Here's how the part is built. I have some questions about the finished solid (model axes, mm). Round coordinates to 2 decimals unless told otherwise and drop trailing zeros. Loops run counter-clockwise (first coordinate to the right, second up) from the corner with the lowest first, then second, coordinate; pieces in that order, holes last. Notation, with made-up numbers: M 10.5,-2.5 L 43.5,-2.5 A15 ccw 43.5,4.5 Z; hole C 75,17 d1. An arc over 180 degrees is marked long. Use a Markdown table: item, result.
```python
from build123d import *

# Parameters (mm, degrees)
SKETCH2_R           = 1
SKETCH2_R_2         = 3
BOSS_EXTRUDE2_DEPTH = 4.7625


with BuildPart() as part:
    # Sketch2 → Boss-Extrude2 (new body)
    # profile 1 of 7: a face of its own
    with BuildSketch(Plane(origin=(0, 0, 0), x_dir=(1, 0, 0), z_dir=(0, 1, 0))):
        with BuildLine():
            Line((0, 32), (0, 30))
            ThreePointArc((0, 30), (21.213203436, 21.213203436), (30, 0))
            Line((30, 0), (33.432819775, 0))
            ThreePointArc((33.432819775, 0), (33.386867146, 5.204755795), (37.902132901, 2.615553276))
            ThreePointArc((37.902132901, 2.615553276), (37.491335421, 1.10028752), (36.371446028, 0))
            Line((36.371446028, 0), (48, 0))
            ThreePointArc((48, 0), (33.941125497, 33.941125497), (0, 48))
            Line((0, 48), (0, 38))
            ThreePointArc((0, 38), (2.121320344, 37.121320344), (3, 35))
            ThreePointArc((3, 35), (2.121320344, 32.878679656), (0, 32))
        make_face()
        with Locations(Location((42.896828136, 9.790921094, 0), (0, 0, 90))):
            Circle(SKETCH2_R, mode=Mode.SUBTRACT)
        with Locations(Location((32.580581203, 12.786935853, 0), (0, 0, 90))):
            Circle(SKETCH2_R_2, mode=Mode.SUBTRACT)
        with Locations(Location((27.364101886, 21.822143065, 0), (0, 0, 90))):
            Circle(SKETCH2_R_2, mode=Mode.SUBTRACT)
        with Locations(Location((10.316431104, 33.445048203, 0), (0, 0, 90))):
            Circle(SKETCH2_R_2, mode=Mode.SUBTRACT)
        with Locations(Location((19.716202032, 28.918357101, 0), (0, 0, 90))):
            Circle(SKETCH2_R_2, mode=Mode.SUBTRACT)
        with Locations(Location((19.090884521, 39.642630188, 0), (0, 0, 90))):
            Circle(SKETCH2_R, mode=Mode.SUBTRACT)
    # profile 2 of 7: a face of its own
    with BuildSketch(Plane(origin=(0, 0, 0), x_dir=(1, 0, 0), z_dir=(0, 1, 0))):
        with BuildLine():
            Line((33.432819775, 0), (30, 0))
            ThreePointArc((30, 0), (0, -30), (-30, 0))
            Line((-30, 0), (-33.432819775, 0))
            ThreePointArc((-33.432819775, 0), (-34.902132901, -0.384446724), (-36.371446028, 0))
            Line((-36.371446028, 0), (-48, 0))
            ThreePointArc((-48, 0), (-44.712414383, -17.458522274), (-35.3, -32.525528435))
            ThreePointArc((-35.3, -32.525528435), (-19.271411924, -43.961490903), (0, -48))
            ThreePointArc((0, -48), (19.271411924, -43.961490903), (35.3, -32.525528435))
            ThreePointArc((35.3, -32.525528435), (44.712414383, -17.458522274), (48, 0))
            Line((48, 0), (36.371446028, 0))
            ThreePointArc((36.371446028, 0), (34.902132901, -0.384446724), (33.432819775, 0))
        make_face()
        with Locations(Location((-34.400585229, -27.433551282, 0), (0, 0, 90))):
            Circle(SKETCH2_R, mode=Mode.SUBTRACT)
        with Locations(Location((-15.185930869, -31.533910377, 0), (0, 0, 90))):
            Circle(SKETCH2_R_2, mode=Mode.SUBTRACT)
        with Locations(Location((-23.806045822, -25.656815514, 0), (0, 0, 90))):
            Circle(SKETCH2_R_2, mode=Mode.SUBTRACT)
        with Locations(Location((-5.216479316, -34.609078918, 0), (0, 0, 90))):
            Circle(SKETCH2_R_2, mode=Mode.SUBTRACT)
        with Locations(Location((-30.310889132, -17.5, 0), (0, 0, 90))):
            Circle(SKETCH2_R_2, mode=Mode.SUBTRACT)
        with Locations(Location((-34.122476926, -7.788232688, 0), (0, 0, 90))):
            Circle(SKETCH2_R_2, mode=Mode.SUBTRACT)
        with Locations(Location((0, -44, 0), (0, 0, 90))):
            Circle(SKETCH2_R, mode=Mode.SUBTRACT)
        with Locations(Location((5.216479316, -34.609078918, 0), (0, 0, 90))):
            Circle(SKETCH2_R_2, mode=Mode.SUBTRACT)
        with Locations(Location((15.185930869, -31.533910377, 0), (0, 0, 90))):
            Circle(SKETCH2_R_2, mode=Mode.SUBTRACT)
        with Locations(Location((23.806045822, -25.656815514, 0), (0, 0, 90))):
            Circle(SKETCH2_R_2, mode=Mode.SUBTRACT)
        with Locations(Location((34.400585229, -27.433551282, 0), (0, 0, 90))):
            Circle(SKETCH2_R, mode=Mode.SUBTRACT)
        with Locations(Location((30.310889132, -17.5, 0), (0, 0, 90))):
            Circle(SKETCH2_R_2, mode=Mode.SUBTRACT)
        with Locations(Location((34.122476926, -7.788232688, 0), (0, 0, 90))):
            Circle(SKETCH2_R_2, mode=Mode.SUBTRACT)
    # profile 3 of 7: a face of its own
    with BuildSketch(Plane(origin=(0, 0, 0), x_dir=(1, 0, 0), z_dir=(0, 1, 0))):
        with BuildLine():
            Line((48, -32.525528435), (48, 0))
            ThreePointArc((48, 0), (44.712414383, -17.458522274), (35.3, -32.525528435))
            Line((35.3, -32.525528435), (48, -32.525528435))
        make_face()
    # profile 4 of 7: a face of its own
    with BuildSketch(Plane(origin=(0, 0, 0), x_dir=(1, 0, 0), z_dir=(0, 1, 0))):
        with BuildLine():
            Line((35.3, -48), (35.3, -32.525528435))
            ThreePointArc((35.3, -32.525528435), (19.271411924, -43.961490903), (0, -48))
            Line((0, -48), (35.3, -48))
        make_face()
    # profile 5 of 7: a face of its own
    with BuildSketch(Plane(origin=(0, 0, 0), x_dir=(1, 0, 0), z_dir=(0, 1, 0))):
        with BuildLine():
            ThreePointArc((0, -48), (-19.271411924, -43.961490903), (-35.3, -32.525528435))
            Line((-35.3, -32.525528435), (-35.3, -48))
            Line((-35.3, -48), (0, -48))
        make_face()
    # profile 6 of 7: a face of its own
    with BuildSketch(Plane(origin=(0, 0, 0), x_dir=(1, 0, 0), z_dir=(0, 1, 0))):
        with BuildLine():
            ThreePointArc((-35.3, -32.525528435), (-44.712414383, -17.458522274), (-48, 0))
            Line((-48, 0), (-48, -32.525528435))
            Line((-48, -32.525528435), (-35.3, -32.525528435))
        make_face()
    # profile 7 of 7: a face of its own
    with BuildSketch(Plane(origin=(0, 0, 0), x_dir=(1, 0, 0), z_dir=(0, 1, 0))):
        with BuildLine():
            ThreePointArc((-30, 0), (-21.213203436, 21.213203436), (0, 30))
            Line((0, 30), (0, 32))
            ThreePointArc((0, 32), (-3, 35), (0, 38))
            Line((0, 38), (0, 48))
            ThreePointArc((0, 48), (-33.941125497, 33.941125497), (-48, 0))
            Line((-48, 0), (-36.371446028, 0))
            ThreePointArc((-36.371446028, 0), (-36.417398657, 5.204755795), (-31.902132901, 2.615553276))
            ThreePointArc((-31.902132901, 2.615553276), (-32.312930381, 1.10028752), (-33.432819775, 0))
            Line((-33.432819775, 0), (-30, 0))
        make_face()
        with Locations(Location((-42.896828136, 9.790921094, 0), (0, 0, 90))):
            Circle(SKETCH2_R, mode=Mode.SUBTRACT)
        with Locations(Location((-32.580581203, 12.786935853, 0), (0, 0, 90))):
            Circle(SKETCH2_R_2, mode=Mode.SUBTRACT)
        with Locations(Location((-27.364101886, 21.822143065, 0), (0, 0, 90))):
            Circle(SKETCH2_R_2, mode=Mode.SUBTRACT)
        with Locations(Location((-19.716202032, 28.918357101, 0), (0, 0, 90))):
            Circle(SKETCH2_R_2, mode=Mode.SUBTRACT)
        with Locations(Location((-10.316431104, 33.445048203, 0), (0, 0, 90))):
            Circle(SKETCH2_R_2, mode=Mode.SUBTRACT)
        with Locations(Location((-19.090884521, 39.642630188, 0), (0, 0, 90))):
            Circle(SKETCH2_R, mode=Mode.SUBTRACT)
    extrude(amount=BOSS_EXTRUDE2_DEPTH)


solid = part.part
```
Q1. Will these pins go through, and if not, where does the flat tip stop? P1, Ø2.5, axis at x = -42, y = 1.5, coming from the +Z side; P2, Ø2, axis at y = 3.5, z = -29, coming from the +X side.
Return value:
| item | result |
|---|---|
| P1 | stops at z = 32.53 |
| P2 | stops at x = 38.99 |
Q2. Imagine slicing it at B-B, the plane z = -23. Please give me the cut outline in (x, y) (1 decimal).
Return value:
| item | result |
|---|---|
| outline | M -42.1,0 L -30.1,0 L -30.1,4.8 L -42.1,4.8 Z; M -24.6,0 L -19.3,0 L -19.3,4.8 L -24.6,4.8 Z; M 19.3,0 L 24.6,0 L 24.6,4.8 L 19.3,4.8 Z; M 30.1,0 L 42.1,0 L 42.1,4.8 L 30.1,4.8 Z |
Q3. Imagine slicing it at C-C, the plane y = 1.25. Give the number of separate pieces and of enclosed holes in the cut face, then the cut area to 3 significant figures.
Return value:
| item | result |
|---|---|
| separate pieces | 1 |
| enclosed holes | 29 |
| area | 4,390 mm^2 |
Q4. We'd pull the mould along X, two halves only. Please class faces 1 (the flat face through (-48, 2, 16)), 2 (the flat face through (35.3, 2, 40)), 3 (the cylindrical face through (30.026, 2.348, -23.206)), 4 (the flat face through (42, 2, 32.526)): pulls with the +X half, pulls with the -X half, needs draft (parallel to the pull), parting line crosses it, or undercut.
Return value:
| item | result |
|---|---|
| face 1 | pulls with the -X half |
| face 2 | pulls with the +X half |
| face 3 | undercut |
| face 4 | needs draft |
Q5. Imagine slicing it at A-A, the plane z = 6. Please give me the cut outline in (x, y).
Return value:
| item | result |
|---|---|
| outline | M -48,0 L -36.53,0 L -36.53,4.76 L -48,4.76 Z; M -31.71,0 L -29.39,0 L -29.39,4.76 L -31.71,4.76 Z; M 29.39,0 L 31.71,0 L 31.71,4.76 L 29.39,4.76 Z; M 36.53,0 L 48,0 L 48,4.76 L 36.53,4.76 Z |
Q6. I need wall thicknesses on line 1 (X direction, y = 2.75, z = 17.5); line 2 (X direction, y = 3.7, z = -2); line 3 (Z direction, x = 2.5, y = 1.3). Which ranges of each line are inside material? Lowest first, please. Write a range as from..to.
Return value:
| item | result |
|---|---|
| line 1 | x = -48..-33.31, -27.31..-24.37, 24.37..27.31, 33.31..48 |
| line 2 | x = -47.96..-37.84, -31.97..-29.93, 29.93..31.97, 37.84..47.96 |
| line 3 | z = -47.93..-36.66, -33.34..-29.9, 29.9..33.34, 35.88..48 |
